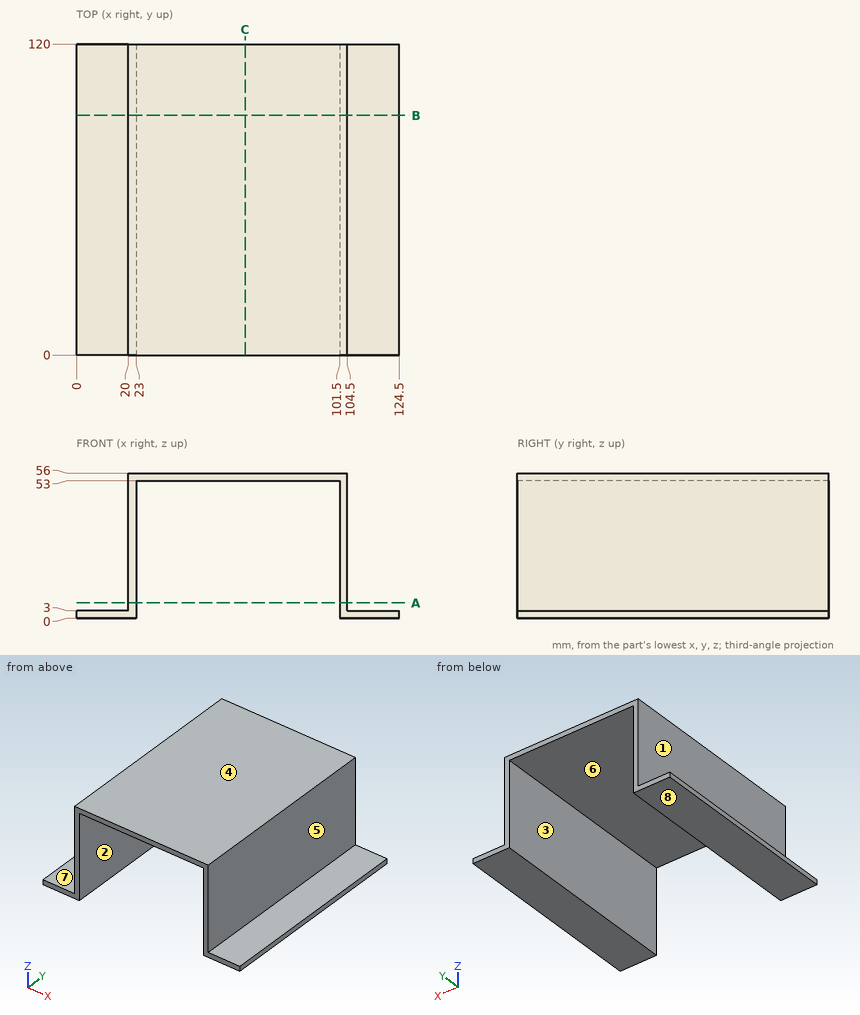
The figure shows three views and two pictorial views of one solid part (mm, origin at its lowest corner). Answer the questions. A direction names the side the tool comes from. Round coordinates to 2 decimals unless told otherwise and drop trailing zeros. Order: outer loops, then holes, each group sorted by start corner. A loop starts at its lowest first (then second) coordinate and runs counter-clockwise, first axis right, second up. Notation, with made-up numbers: M -1,32.25 L 32,32.25 A11 ccw 32,53.25 Z; hole C 19,14 d2. An arc over 180 degrees is marked long. Answer in a Markdown table with one row per item. Add a question column.
1) Consider line 1 along X through (y, z) = (71, 44); line 2 along Z through (x, y) = (109.5, 101); line 3 along Z through (x, y) = (38.5, 49). Determine where each line is inside the solid, lowest interval first. Write a range as from..to.
2) The part is cut by section B-B on y = 92.5. Determine the outline of the cut face in (x, z), plus the area to 4 significant figures.
3) The part is cut by section A-A on z = 6. Determine the outline of the cut face in (x, y).
4) The part is cut by section C-C on x = 65. Determine the outline of the cut face in (y, z).
5) Which of the six approach directions +Z, -Z, +X, -X, +Y, -Y give full straight-line access (tool end or side, diameter ignored) to the marked faces 5, 6, 7 and 8?
6) Flat-ended cylindrical pins translate along their axes: pin 1 Ø6 at (x, y) = (117, 72.5) entering from +Z; pin 2 Ø2 at (y, z) = (20.5, 15) entering from +X; pin 3 Ø4 at (x, y) = (48, 67.5) entering from -Z. Find the tip coordinate at first contact, or state that the pin passes through.
7) Determine the mould class of the marked faces 1, 2, 3 and 4 for opening direction X: pulls with the +X half, pulls with the -X half, needs draft (parallel to the pull), parting line crosses it, or undercut.
Findings below:
| question | item | result |
|---|---|---|
| 1 | line 1 | x = 20..23, 101.5..104.5 |
| 1 | line 2 | z = 0..3 |
| 1 | line 3 | z = 53..56 |
| 2 | outline | M 0,0 L 23,0 L 23,53 L 101.5,53 L 101.5,0 L 124.5,0 L 124.5,3 L 104.5,3 L 104.5,56 L 20,56 L 20,3 L 0,3 Z |
| 2 | area | 691.5 mm² |
| 3 | outline | M 20,0 L 23,0 L 23,120 L 20,120 Z; M 101.5,0 L 104.5,0 L 104.5,120 L 101.5,120 Z |
| 4 | outline | M 0,53 L 120,53 L 120,56 L 0,56 Z |
| 5 | face 5 | +Z, +X, +Y, -Y |
| 5 | face 6 | -Z, +Y, -Y |
| 5 | face 7 | +Z, -X, +Y, -Y |
| 5 | face 8 | -Z, +X, -X, +Y, -Y |
| 6 | pin 1 | stops at z = 3 |
| 6 | pin 2 | stops at x = 104.5 |
| 6 | pin 3 | stops at z = 53 |
| 7 | face 1 | pulls with the -X half |
| 7 | face 2 | undercut |
| 7 | face 3 | undercut |
| 7 | face 4 | needs draft |
